from build123d import *

# Parameters (mm, degrees)
F0_R         = 18.3771927797
F1_DEPTH     = 89.916
F2_R         = 53.2482574965
F2_R_2       = 18.3771927797
F3_DEPTH     = 5.588
F5_S5_R      = 53.2482574965
F5_T6_DEPTH  = 79
F5_S11_R     = 53.2482574965
F5_T12_DEPTH = 79


# Not quite as in the source:
# - a fillet or chamfer that OpenCascade refuses, or shapes differently, is made with other operations: its cross-section is extruded or revolved along the edge and cut away or added


with BuildPart() as f1:
    # F0 (on Top) → F1 (new body)
    with BuildSketch(Plane.XY):
        Circle(F0_R)
    extrude(amount=F1_DEPTH)

    # F2 (on face) → F3 (join)
    with BuildSketch(Plane.XY.offset(89.916)):
        Circle(F2_R)
        Circle(F2_R_2, mode=Mode.SUBTRACT)
        Circle(F2_R_2)
    extrude(amount=F3_DEPTH)

    # F4: F1 across plane


with BuildPart() as f1_1:
    add(f1.part)
    add(f1.part.mirror(Plane.XY))

    # F5: chamfer of 35.306 on 5 edges, made by hand


with BuildPart() as f5_tool2:
    # F5_s3 → F5_t4 (revolve)
    with BuildSketch(Plane.XZ):
        Polygon((53.6831927797, 89.916), (18.3771927797, 54.61), (18.3771927797, 89.916), align=None)
    revolve(axis=Axis((0, 0, 89.916), (0, 0, 1)))

    # F5_s5 → F5_t6 (intersect, symmetric)
    with BuildSketch(Plane.XY.offset(72.3)):
        Circle(F5_S5_R)
    extrude(amount=F5_T6_DEPTH, both=True, mode=Mode.INTERSECT)


with BuildPart() as f1_2:
    add(f1_1.part)

    # F5_t1: union F5_tool2
    add(f5_tool2.part)


with BuildPart() as f5_tool8:
    # F5_s9 → F5_t10 (revolve)
    with BuildSketch(Plane.XZ):
        Polygon((18.3771927797, -54.61), (53.6831927797, -89.916), (18.3771927797, -89.916), align=None)
    revolve(axis=Axis((0, 0, -89.916), (0, 0, 1)))

    # F5_s11 → F5_t12 (intersect, symmetric)
    with BuildSketch(Plane.XY.offset(-72.3)):
        Circle(F5_S11_R)
    extrude(amount=F5_T12_DEPTH, both=True, mode=Mode.INTERSECT)


with BuildPart() as f1_3:
    add(f1_2.part)

    # F5_t7: union F5_tool8
    add(f5_tool8.part)


solid = f1_3.part
The listing builds one solid part. Answer for the finished solid, in the listing's coordinates (mm). A direction names the side the tool comes from. Round coordinates to 2 decimals unless told otherwise and drop trailing zeros. Write each loop counter-clockwise with the first axis right and the second up, starting at its lowest first coordinate (ties: lowest second). Pieces come first, ordered by that corner, then holes. Notation, with made-up numbers: M -13.5,-2.75 L 7.5,-2.75 A20 ccw 7.5,33.25 Z; hole C 25.5,-27.5 d3. An arc over 180 degrees is marked long. Write each question's results on one line, items separated by ' | '. Start each with the question number.
Item 1: Straight lines are drawn through the part: L1, parallel to Z at x = -0.5, y = -34; L2, parallel to Z at x = 16, y = 10; L3, parallel to X at y = 1, z = -31. For each, find the intervals that lie inside material, in ascending order. Write a range as [from, to].
Item 2: Flat-ended cylindrical pins translate along their axes: pin 1 Ø4 at (x, z) = (11, -62) entering from +Y; pin 2 Ø12 at (x, z) = (8, 6.5) entering from +Y; pin 3 Ø1.5 at (y, z) = (14, 49) entering from -X. Find the tip coordinate at first contact, or state that the pin passes through.
Item 3: For faces 5 (the face through (19.14, 6.03, 56.3)), 6 (the face through (50.79, 15.99, -92.45)), determine the directions among +Z, -Z, +X, -X, +Y, -Y from which every point of the face is accessible in a straight line to the end or side of a thin tool.
Item 4: For a pull along Z with two mould halves and no side action, classify faces 1 (the face through (19.609, 6.175, -56.791)), 2 (the face through (50.79, 15.99, 92.53)), 3 (the face through (-1, 1, 95.504)), 4 (the face through (-1, 1, -95.504)) as pulls with the +Z half, pulls with the -Z half, needs draft (parallel to the pull), parting line crosses it, or undercut.
Item 5: A cutting plane is placed at A-A on y = 0. Write down the section's boundary in (x, z), and give its area (3 significant figures).
Item 6: A cutting plane is placed at C-C on z = -48.5. Write down the section's boundary in (x, y).
Item 7: A cutting plane is placed at D-D on z = 73. Write down the section's boundary in (x, y), and give its area (3 significant figures).
Check sheet entries:
1) L1: [-95.5, -70.24], [70.24, 95.5] | L2: [-95.5, -55.1], [55.1, 95.5] | L3: [-18.35, 18.35]
2) pin 1: y = 25.65 | pin 2: y = 18.27 | pin 3: x = -12.73
3) face 5: none | face 6: +Z, -Z
4) face 1: undercut | face 2: needs draft | face 3: pulls with the +Z half | face 4: pulls with the -Z half
5) outline: M -53.25,-95.5 L 53.25,-95.5 L 53.25,-89.48 L 18.38,-54.61 L 18.38,54.61 L 53.25,89.48 L 53.25,95.5 L -53.25,95.5 L -53.25,89.48 L -18.38,54.61 L -18.38,-54.61 L -53.25,-89.48 Z | area: 10,300 mm²
6) outline: C 0,0 d36.75
7) outline: C 0,0 d73.53 | area: 4,250 mm²
